Input: dimensioned drawing with shaded views. Units: mm. Origin: part minimum x, y, z. Round coordinates to 2 decimals unless told otherwise and drop trailing zeros. Order: outer loops, then holes, each group sorted by start corner. A loop starts at its lowest first (then second) coordinate and runs counter-clockwise, first axis right, second up.
Item 1: Mould query, pull axis Z, two halves, no side actions, for the marked faces 1, 2 and 3. Classes: released by +Z, released by -Z, zero draft, split by the parting line, or undercut.
Item 2: Cut plane A-A on y = 31.75. Give the number of separate pieces and of enclosed holes in the cut face, then the cut area to 3 significant figures.
Item 3: Cut plane B-B on z = 88.9. Output: boundary loops of the cut face in (x, y), then the cut area to 3 significant figures.
Item 4: Line query: L1, parallel to Z at x = 7, y = 11 (1 decimal); L2, parallel to Z at x = 8.75, y = 10 (1 decimal); L3, parallel to Z at x = 5.25, y = 17.5 (1 decimal). Output: solid intervals per line, ascending.
Item 5: Cut plane D-D on z = 50.8. Output: boundary loops of the cut face in (x, y) (1 decimal), then the cut area to 3 significant figures.
Item 6: First-contact query: pin 1 (4 mm diameter, centred on x = 8, z = 12.5, fed in from +Y); pin 2 (5.5 mm diameter, centred on x = 6.35, z = 12.7, fed in from -Y); pin 3 (4 mm diameter, centred on x = 8.5, z = 70, fed in from -Y) (1 decimal); pin 4 (6 mm diameter, centred on x = 5, z = 55.5, fed in from -Y). Flat tips, straight axial feed; report the tip coordinate or a pass-through.
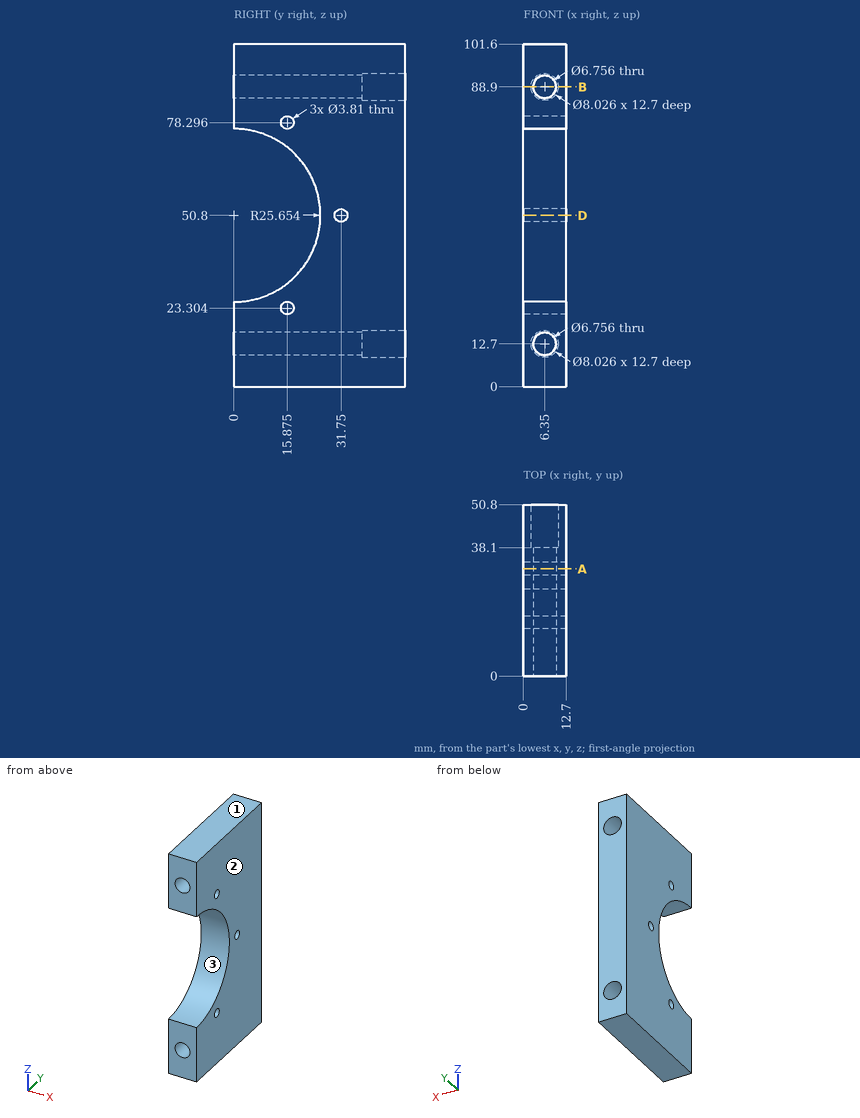
From the geometry:
1. face 1: released by +Z
1. face 2: zero draft
1. face 3: undercut
2. separate pieces: 2
2. enclosed holes: 2
2. area: 1,170 mm2
3. outline: (0, 0) - (2.97, 0) - (2.97, 38.1) - (2.34, 38.1) - (2.34, 50.8) - (0, 50.8) - close; (9.73, 0) - (12.7, 0) - (12.7, 50.8) - (10.36, 50.8) - (10.36, 38.1) - (9.73, 38.1) - close
3. area: 286 mm2
4. L1: z = 0 to 9.4, 16 to 27.6, 74 to 85.6, 92.2 to 101.6
4. L2: z = 0 to 10.3, 15.1 to 27.2, 74.4 to 86.5, 91.3 to 101.6
4. L3: z = 0 to 9.5, 15.9 to 22.3, 24.3 to 32, 69.6 to 77.3, 79.3 to 85.7, 92.1 to 101.6
5. outline: (0, 25.7) - (12.7, 25.7) - (12.7, 29.8) - (0, 29.8) - close; (0, 33.7) - (12.7, 33.7) - (12.7, 50.8) - (0, 50.8) - close
5. area: 271 mm2
6. pin 1: stops at y = 38.1
6. pin 2: passes through
6. pin 3: stops at y = 14.4
6. pin 4: stops at y = 24.47
